from build123d import *

# Parameters (mm, degrees)
SKETCH_1_W          = 7
SKETCH_1_H          = 7
EXTRUDE_1_DEPTH     = 107
FILLET_1_R          = 3.5
SKETCH_5_R          = 1.55
CUT_EXTRUDE_2_DEPTH = 108.285833175
SKETCH_6_W          = 7
SKETCH_6_H          = 3
EXTRUDE_2_DEPTH     = 7
FILLET_2_R          = 3.5
SKETCH_7_R          = 1.55
CUT_EXTRUDE_4_DEPTH = 105.587284122
FILLET_3_R          = 1.5
FILLET_4_R          = 0.8
FILLET_5_R          = 0.8


# Some blends are built 0.0001 mm under size
with BuildPart() as part:
    # 草图1 → 凸台-拉伸1 (new body)
    with BuildSketch(Plane.XY):
        Rectangle(SKETCH_1_W, SKETCH_1_H)
    extrude(amount=EXTRUDE_1_DEPTH)

    # 圆角1
    fillet_1_edges = [part.edges().sort_by_distance(p)[0] for p in [
        (0, -3.5, 107),
    ]]
    fillet(fillet_1_edges, radius=FILLET_1_R)

    # 草图5 → 切除-拉伸2 (cut, through all)
    with BuildSketch(Plane(origin=(3.5, 0, 0), x_dir=(0, 0, -1), z_dir=(1, 0, 0))):
        with Locations(Location((-103.5, 0, 0), (0, 0, 90))):
            Circle(SKETCH_5_R)
    extrude(amount=-CUT_EXTRUDE_2_DEPTH, mode=Mode.SUBTRACT)

    # 草图6 → 凸台-拉伸2 (add)
    with BuildSketch(Plane(origin=(0, 3.5, 0), x_dir=(1, 0, 0), z_dir=(0, 1, 0))):
        with Locations((0, -105.5)):
            Rectangle(SKETCH_6_W, SKETCH_6_H)
    extrude(amount=EXTRUDE_2_DEPTH)

    # 圆角2
    fillet_2_edges = [part.edges().sort_by_distance(p)[0] for p in [
        (3.5, 10.5, 105.5),
        (-3.5, 10.5, 105.5),
    ]]
    fillet(fillet_2_edges, radius=FILLET_2_R - 0.0001)  # a hair under: the kernel refuses the full size

    # 草图7 → 切除-拉伸4 (cut, through all)
    with BuildSketch(Plane(origin=(0, 0, 104), x_dir=(-1, 0, 0), z_dir=(0, 0, -1))):
        with Locations((0, 7)):
            Circle(SKETCH_7_R)
    extrude(amount=-CUT_EXTRUDE_4_DEPTH, mode=Mode.SUBTRACT)

    # 圆角3
    fillet_3_edges = [part.edges().sort_by_distance(p)[0] for p in [
        (0, 3.5, 104),
    ]]
    fillet(fillet_3_edges, radius=FILLET_3_R)

    # 圆角4
    fillet_4_edges = [part.edges().sort_by_distance(p)[0] for p in [
        (-3.5, 6.00005, 104),
        (3.5, 6.00005, 104),
        (-2.474903023, 9.474903023, 104),
        (2.474903023, 9.474903023, 104),
        (3.5, 3.5, 51.25),
        (-3.5, 3.5, 51.25),
        (-3.5, 3.939339828, 103.560660172),
        (3.5, 3.939339828, 103.560660172),
    ]]
    fillet(fillet_4_edges, radius=FILLET_4_R)

    # 圆角5
    # the kernel refuses this fillet: 0.8 mm, written as the material it takes off along each edge
    with BuildSketch(Plane(origin=(3.5, -3.5, -4.8), x_dir=(0, 1, 0), z_dir=(0, 0, 1)), Plane(origin=(-3.5, -3.5, -4.8), x_dir=(1, 0, 0), z_dir=(0, 0, 1))) as fillet_5_piece_1:
        with BuildLine():
            CenterArc((FILLET_5_R, FILLET_5_R), FILLET_5_R, 180, 90)
            Line((0, FILLET_5_R), (-FILLET_5_R * 0.02, FILLET_5_R))
            Line((-FILLET_5_R * 0.02, FILLET_5_R), (-FILLET_5_R * 0.02, -FILLET_5_R * 0.02))
            Line((-FILLET_5_R * 0.02, -FILLET_5_R * 0.02), (FILLET_5_R, -FILLET_5_R * 0.02))
            Line((FILLET_5_R, -FILLET_5_R * 0.02), (FILLET_5_R, 0))
        make_face()
    extrude(amount=113.1, mode=Mode.SUBTRACT)


solid = part.part
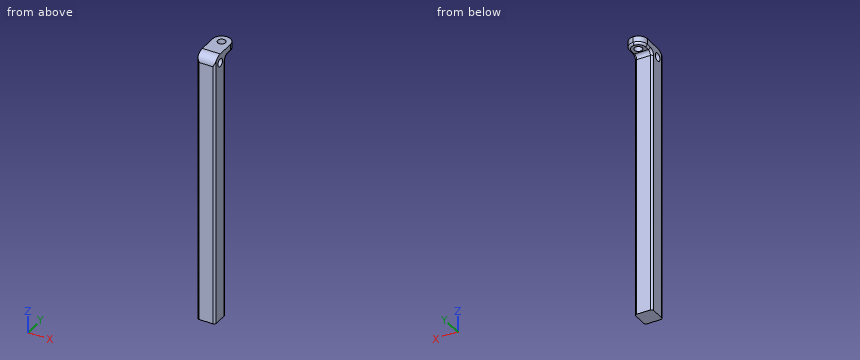
Here's how the part is built. I have some questions about the finished solid (model axes, mm). Coordinates: 2 decimals unless noted, no trailing zeros. Order: outer loops, then holes, each group sorted by start corner. A loop starts at its lowest first (then second) coordinate and runs counter-clockwise, first axis right, second up. Notation, with made-up numbers: M 17.5,82.25 L 61.5,82.25 A16 ccw 61.5,106.25 Z; hole C -38.75,-22.75 d10. An arc over 180 degrees is marked long. Answer as CSV lines item,"result". Start each with the question number.
1. I need wall thicknesses on line 1 (Z direction, x = -1.5, y = 0); line 2 (Y direction, x = 1, z = 96); line 3 (Z direction, x = 0.75, y = 8.5). Which ranges of each line are inside material? Lowest first, please. Write a range as [from, to].
2. For pin 1 (2.5 mm diameter, centred on y = 0, z = 103.5, fed in from +X); pin 2 (2.5 mm diameter, centred on x = -1, y = 8.5, fed in from -Z), each with a flat end and sliding along its axis, tell me the tip position at first contact or that it passes through.
3. I want a section at A-A, the plane z = 27.5. Write out the boundary of the cut face in (x, y).
Recorded:
1,line 1,"z = [0, 101.95], [105.05, 107]"
1,line 2,"y = [-3.5, 3.5]"
1,line 3,"z = [104, 107]"
2,pin 1,"passes through"
2,pin 2,"stops at z = 104"
3,outline,"M -3.5,-2.7 A0.8 ccw -2.7,-3.5 L 2.7,-3.5 A0.8 ccw 3.5,-2.7 L 3.5,2.7 A0.8 ccw 2.7,3.5 L -2.7,3.5 A0.8 ccw -3.5,2.7 Z"
